Here's the drawing with two shaded views (mm, measured from the low corner). I have some questions. A direction names the side the tool comes from. Round coordinates to 2 decimals unless told otherwise and drop trailing zeros. Loops run counter-clockwise (first coordinate to the right, second up) from the corner with the lowest first, then second, coordinate; pieces in that order, holes last.
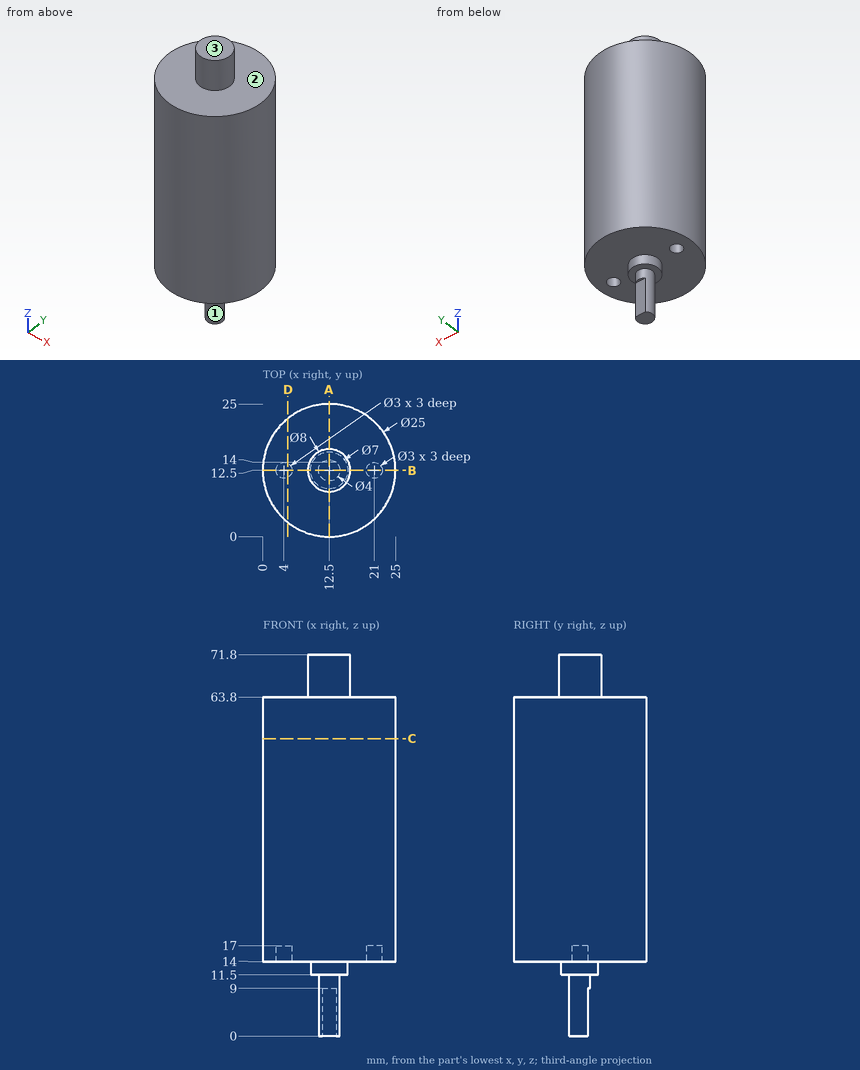
(1) If we section it at A-A, the plane x = 12.5: List the corners of the cut face in (y, z) for me, then the cut area to 3 significant figures.
Worked answers:
outline: (0, 14) - (9, 14) - (9, 11.5) - (10.5, 11.5) - (10.5, 0) - (14, 0) - (14, 9) - (14.5, 9) - (14.5, 11.5) - (16, 11.5) - (16, 14) - (25, 14) - (25, 63.8) - (16.5, 63.8) - (16.5, 71.8) - (8.5, 71.8) - (8.5, 63.8) - (0, 63.8) - close
area: 1,370 mm2
(2) If I drill on line 1 (Z direction, x = 15.75, y = 14.75); line 2 (Z direction, x = 17.5, y = 15.25); line 3 (Y direction, x = 4, z = 16.15), over which ranges is the centre line in solid material (lowest first)?
Worked answers:
line 1: z = 14 to 71.8
line 2: z = 14 to 63.8
line 3: y = 3.33 to 11, 14 to 21.67
(3) Will these pins go through, and if not, where does the flat tip stop? P1, Ø1.5, axis at x = 4, y = 12.5, coming from the -Z side; P2, Ø5, axis at y = 4.5, z = 17, coming from the -X side (3 decimals); P3, Ø6, axis at x = 18.5, z = 44.5, coming from the +Y side.
Worked answers:
P1: stops at z = 17
P2: stops at x = 1.275
P3: stops at y = 24.63
(4) For the marked faces 1, 2 and 3, which set-ups out of +Z, -Z, +X, -X, +Y, -Y let a thin tool reach every point of the face, with its end or its side?
Worked answers:
face 1: -Z
face 2: +Z
face 3: +Z, +X, -X, +Y, -Y
(5) If we section it at D-D, the plane x = 4.75: List the corners of the cut face in (y, z) for me.
Worked answers:
outline: (2.69, 14) - (11.2, 14) - (11.2, 17) - (13.8, 17) - (13.8, 14) - (22.31, 14) - (22.31, 63.8) - (2.69, 63.8) - close
(6) If we section it at C-C, the plane z = 56: List the corners of the cut face in (x, y) for me, then the cut area to 3 significant figures.
Worked answers:
outline: circle Ø25 at (12.5, 12.5)
area: 491 mm2
(7) If we section it at B-B, the plane y = 12.5: List the corners of the cut face in (x, z) for me, then the cut area to 3 significant figures.
Worked answers:
outline: (0, 14) - (2.5, 14) - (2.5, 17) - (5.5, 17) - (5.5, 14) - (9, 14) - (9, 11.5) - (10.5, 11.5) - (10.5, 0) - (14.5, 0) - (14.5, 11.5) - (16, 11.5) - (16, 14) - (19.5, 14) - (19.5, 17) - (22.5, 17) - (22.5, 14) - (25, 14) - (25, 63.8) - (16.5, 63.8) - (16.5, 71.8) - (8.5, 71.8) - (8.5, 63.8) - (0, 63.8) - close
area: 1,350 mm2
